The listing builds one solid part. Answer for the finished solid, in the listing's coordinates (mm). Round coordinates to 2 decimals unless told otherwise and drop trailing zeros. Order: outer loops, then holes, each group sorted by start corner. A loop starts at its lowest first (then second) coordinate and runs counter-clockwise, first axis right, second up. Notation, with made-up numbers: M -33.5,66 L -19.5,66 A22 cw -19.5,102 Z; hole C 6,-34 d2. An arc over 180 degrees is marked long. Write item = value, one per line. Start each with the question number.
(1) A cutting plane is placed at D-D, the plane x = -2.25. Determine the outline of the cut face in (y, z).
(2) A cutting plane is placed at C-C, the plane x = 5. Determine the outline of the cut face in (y, z), and give its area (3 significant figures).
(3) A cutting plane is placed at B-B, the plane z = 7.5. Determine the outline of the cut face in (x, y), and give its area (3 significant figures).
(4) Each of these flat-tipped pins is pushed along its axis until it touches: pin 1 (2.5 mm diameter, centred on x = 0, y = 15, fed in from -Z); pin 2 (4 mm diameter, centred on y = 11.5, z = 1.5, fed in from -X); pin 3 (7 mm diameter, centred on x = -3, y = 7.5, fed in from +Z); pin 4 (0.8 mm diameter, centred on x = -0.5, z = 0.5, fed in from +Y). Where does it stop, or does it pass through?
(5) Straight lines are drawn through the part: probe 1 along Y at (x, z) = (-7.5, 0.5); probe 2 along Z at (x, y) = (3.25, -15.5); probe 3 along X at (y, z) = (-15, 0.6). For each, find the intervals that lie inside material, in ascending order. Write a range as from..to.
(6) A cutting plane is placed at A-A, the plane x = -7.5. Determine the outline of the cut face in (y, z).
from build123d import *

# Parameters (mm, degrees)
F1_DEPTH  = 1
F2_DEPTH  = 4
F3_DEPTH  = 4
F4_R      = 0.55
F5_DEPTH  = 4
F6_R      = 0.55
F7_DEPTH  = 4
F8_R      = 0.55
F9_DEPTH  = 4
F10_R     = 0.55
F11_DEPTH = 4


with BuildPart() as f1:
    # F0 (on Top) → F1 (new body)
    with BuildSketch(Plane.XY):
        with BuildLine():
            Line((-6.5, -20), (6.5, -20))
            ThreePointArc((6.5, -20), (6.660315, -19.456926), (7.089859, -19.087978))
            ThreePointArc((7.089859, -19.087978), (3.1, 0), (7.089859, 19.087978))
            ThreePointArc((7.089859, 19.087978), (6.660315, 19.456926), (6.5, 20))
            Line((6.5, 20), (-6.5, 20))
            ThreePointArc((-6.5, 20), (-6.660315, 19.456926), (-7.089859, 19.087978))
            ThreePointArc((-7.089859, 19.087978), (-3.1, 0), (-7.089859, -19.087978))
            ThreePointArc((-7.089859, -19.087978), (-6.660315, -19.456926), (-6.5, -20))
        make_face()
        with BuildLine():
            ThreePointArc((1.5, -15), (-1.06066, -16.06066), (0, -13.5))
            ThreePointArc((0, -13.5), (1.06066, -13.93934), (1.5, -15))
        make_face(mode=Mode.SUBTRACT)
        with BuildLine():
            ThreePointArc((1.5, 15), (1.06066, 13.93934), (0, 13.5))
            ThreePointArc((0, 13.5), (-1.06066, 16.06066), (1.5, 15))
        make_face(mode=Mode.SUBTRACT)
    extrude(amount=F1_DEPTH)

    # F0 (on Top) → F2 (join)
    with BuildSketch(Plane.XY):
        with BuildLine():
            ThreePointArc((6.5, 20), (6.660315, 19.456926), (7.089859, 19.087978))
            ThreePointArc((7.089859, 19.087978), (8.043074, 19.160315), (8.5, 20))
            ThreePointArc((8.5, 20), (7.5, 21), (6.5, 20))
        make_face()
    extrude(amount=F2_DEPTH)

    # F0 (on Top) → F3 (join)
    with BuildSketch(Plane.XY):
        with BuildLine():
            ThreePointArc((-6.5, 20), (-8.339685, 20.543074), (-7.089859, 19.087978))
            ThreePointArc((-7.089859, 19.087978), (-6.660315, 19.456926), (-6.5, 20))
        make_face()
        with BuildLine():
            ThreePointArc((7.089859, -19.087978), (6.660315, -19.456926), (6.5, -20))
            ThreePointArc((6.5, -20), (7.5, -21), (8.5, -20))
            ThreePointArc((8.5, -20), (8.043074, -19.160315), (7.089859, -19.087978))
        make_face()
        with BuildLine():
            ThreePointArc((-7.089859, -19.087978), (-8.339685, -20.543074), (-6.5, -20))
            ThreePointArc((-6.5, -20), (-6.660315, -19.456926), (-7.089859, -19.087978))
        make_face()
    extrude(amount=F3_DEPTH)

    # F4 (on face) → F5 (join)
    with BuildSketch(Plane.XY.offset(4)):
        with Locations((7.5, 20)):
            Circle(F4_R)
    extrude(amount=F5_DEPTH)

    # F6 (on face) → F7 (join)
    with BuildSketch(Plane.XY.offset(4)):
        with Locations((-7.5, 20)):
            Circle(F6_R)
    extrude(amount=F7_DEPTH)

    # F8 (on face) → F9 (join)
    with BuildSketch(Plane.XY.offset(4)):
        with Locations((7.5, -20)):
            Circle(F8_R)
    extrude(amount=F9_DEPTH)

    # F10 (on face) → F11 (join)
    with BuildSketch(Plane.XY.offset(4)):
        with Locations((-7.5, -20)):
            Circle(F10_R)
    extrude(amount=F11_DEPTH)


solid = f1.part
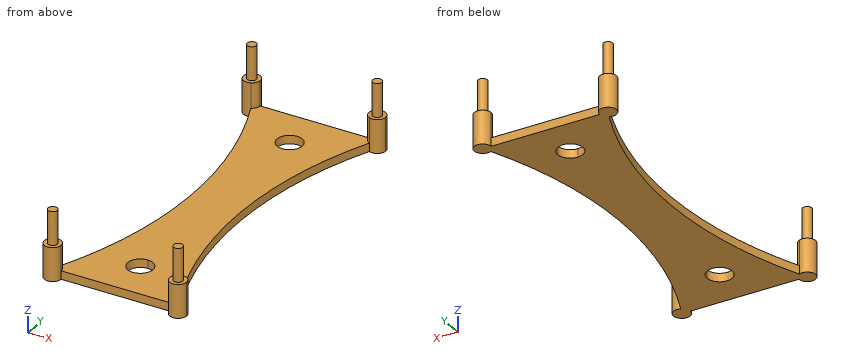
Reported:
q1.outline = M -20,0 L 20,0 L 20,1 L -20,1 Z
q2.outline = M -20,0 L -13.32,0 L -13.32,1 L -20,1 Z; M 13.32,0 L 20,0 L 20,1 L 13.32,1 Z
q2.area = 13.4 mm²
q3.outline = C -7.5,-20 d1.1; C -7.5,20 d1.1; C 7.5,-20 d1.1; C 7.5,20 d1.1
q3.area = 3.80 mm²
q4.pin_1 = through
q4.pin_2 = -5.03
q4.pin_3 = 1
q4.pin_4 = 20
q5.probe_1 = -21..-19, 19..21
q5.probe_2 = 0..1
q5.probe_3 = -5.52..-1.5, 1.5..5.52
q6.outline = M -21,0 L -19,0 L -19,4 L -19.45,4 L -19.45,8 L -20.55,8 L -20.55,4 L -21,4 Z; M 19,0 L 21,0 L 21,4 L 20.55,4 L 20.55,8 L 19.45,8 L 19.45,4 L 19,4 Z
